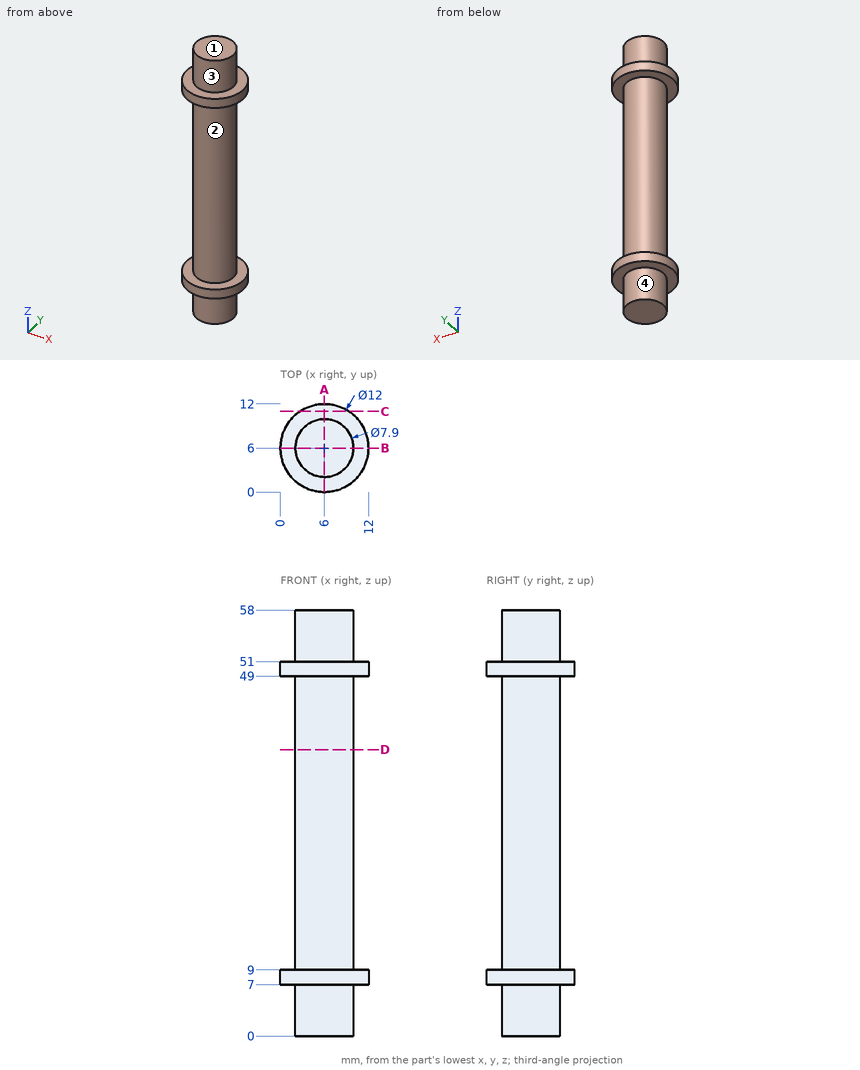
Geometry check sheet. Reference: drawing and pictorial views, mm from the part's lowest x, y, z. A direction names the side the tool comes from. Give positions to 0.01 mm unless a question says otherwise; leave off trailing zeros. Order: outer loops, then holes, each group sorted by start corner. A loop starts at its lowest first (then second) coordinate and runs counter-clockwise, first axis right, second up.
1. Gauge pin test, flat ends, axial feed: pin 1 Ø3 at (x, z) = (4.5, 31) entering from +Y; pin 2 Ø5 at (x, z) = (8.5, 24) entering from -Y. Record the tip position at first contact, or that the pin passes through.
2. Section check C-C, the plane y = 11. Enter the section's corners in (x, z), and give its area (3 significant figures).
3. Thickness scan on L1, parallel to Z at x = 7.25, y = 10; L2, parallel to Y at x = 5.75, z = 3; L3, parallel to X at y = 5, z = 25.5. Record the ranges inside material, lowest first.
4. Section check D-D, the plane z = 39. Enter the section's corners in (x, y).
5. Section check A-A, the plane x = 6. Enter the section's corners in (y, z).
6. Access from +Z, -Z, +X, -X, +Y, -Y to the whole of each face (thin tool, end or side, straight path). Record for the marked faces 1, 2, 3 and 4.
Values follow:
1. pin 1: stops at y = 9.95
1. pin 2: stops at y = 2.05
2. outline: (2.68, 7) - (9.32, 7) - (9.32, 9) - (2.68, 9) - close; (2.68, 49) - (9.32, 49) - (9.32, 51) - (2.68, 51) - close
2. area: 26.5 mm2
3. L1: z = 7 to 9, 49 to 51
3. L2: y = 2.06 to 9.94
3. L3: x = 2.18 to 9.82
4. outline: circle Ø7.9 at (6, 6)
5. outline: (0, 7) - (2.05, 7) - (2.05, 0) - (9.95, 0) - (9.95, 7) - (12, 7) - (12, 9) - (9.95, 9) - (9.95, 49) - (12, 49) - (12, 51) - (9.95, 51) - (9.95, 58) - (2.05, 58) - (2.05, 51) - (0, 51) - (0, 49) - (2.05, 49) - (2.05, 9) - (0, 9) - close
6. face 1: +Z, +X, -X, +Y, -Y
6. face 2: none
6. face 3: +Z
6. face 4: -Z
